Work out the finished part from the listing and answer in its coordinate system (mm). A direction names the side the tool comes from. Round coordinates to 2 decimals unless told otherwise and drop trailing zeros. Order: outer loops, then holes, each group sorted by start corner. A loop starts at its lowest first (then second) coordinate and runs counter-clockwise, first axis right, second up. Notation, with made-up numbers: (-22.75, 51.5) -> (3.25, 51.5) arc R19 ccw to (3.25, 73.5) -> close; hole circle Ø11 at (42.5, 2.25). An arc over 180 degrees is marked (long way). Use a Markdown table: item, result. Add a question column.
Item 1: A cutting plane is placed at A-A, the plane x = -8.25. Determine the outline of the cut face in (y, z), plus the area to 3 significant figures.
Item 2: A tool of negligible diameter and unlimited length cuts with its end or side. For faces 1 (the flat face through (-6, -131, 12.7)), 2 (the flat face through (-6, -131, 10.16)), from which of +Z, -Z, +X, -X, +Y, -Y can it reach the whole face along a straight path? Write none if from no direction.
Item 3: A cutting plane is placed at B-B, the plane z = 8.25. Determine the outline of the cut face in (x, y).
Item 4: A cutting plane is placed at C-C, the plane y = -51. Determine the outline of the cut face in (x, z).
Item 5: For a pull along X with two mould halves and no side action, classify faces 3 (the flat face through (0, -131, 6)), 4 (the flat face through (-2, 0, 6)), 5 (the flat face through (-2.54, -131, 6)) as +X half, -X half, draft (parallel to the pull), parting line (faces both ways), or undercut.
Item 6: Find the intervals of material crossed by L1, parallel to Z at x = -10, y = -123; L2, parallel to X at y = -116, z = 5, in increasing order. Write a range as [from, to].
from build123d import *

# Parameters (mm, degrees)
F0_W     = 7.62
F0_H     = 7.62
F1_DEPTH = 265.43


with BuildPart() as f1:
    # F0 (on Front) → F1 (new body)
    with BuildSketch(Plane.XZ):
        Polygon((-12.7, 0), (0, 0), (0, 12.7), (-10.16, 12.7), (-12.7, 12.7), align=None)
        with Locations((-6.35, 6.35)):
            Rectangle(F0_W, F0_H, mode=Mode.SUBTRACT)
    extrude(amount=F1_DEPTH)


solid = f1.part
Reported:
| question | item | result |
|---|---|---|
| 1 | outline | (-265.43, 0) -> (0, 0) -> (0, 2.54) -> (-265.43, 2.54) -> close; (-265.43, 10.16) -> (0, 10.16) -> (0, 12.7) -> (-265.43, 12.7) -> close |
| 1 | area | 1,350 mm² |
| 2 | face 1 | +Z, +X, -X, +Y, -Y |
| 2 | face 2 | +Y, -Y |
| 3 | outline | (-12.7, -265.43) -> (-10.16, -265.43) -> (-10.16, 0) -> (-12.7, 0) -> close; (-2.54, -265.43) -> (0, -265.43) -> (0, 0) -> (-2.54, 0) -> close |
| 4 | outline | (-12.7, 0) -> (0, 0) -> (0, 12.7) -> (-12.7, 12.7) -> close; hole (-10.16, 2.54) -> (-2.54, 2.54) -> (-2.54, 10.16) -> (-10.16, 10.16) -> close |
| 5 | face 3 | +X half |
| 5 | face 4 | draft |
| 5 | face 5 | undercut |
| 6 | L1 | [0, 2.54], [10.16, 12.7] |
| 6 | L2 | [-12.7, -10.16], [-2.54, 0] |
